```python
from build123d import *

# Parameters (mm, degrees)
SKETCH1_W           = 38.1
SKETCH1_H           = 15.24
BOSS_EXTRUDE2_DEPTH = 30.48
SKETCH2_W           = 50.8
SKETCH2_H           = 15.24
BOSS_EXTRUDE3_DEPTH = 38.1
SKETCH3_W           = 38.1
SKETCH3_H           = 17.78
CUT_EXTRUDE1_DEPTH  = 75.703641143
FILLET1_R           = 5.08
FILLET2_R           = 7.62


with BuildPart() as part:
    # Sketch1 → Boss-Extrude2 (new body)
    with BuildSketch(Plane.XY):
        Rectangle(SKETCH1_W, SKETCH1_H)
    extrude(amount=BOSS_EXTRUDE2_DEPTH)

    # Sketch2 → Boss-Extrude3 (add)
    with BuildSketch(Plane.XY.offset(30.48)):
        Rectangle(SKETCH2_W, SKETCH2_H)
    extrude(amount=BOSS_EXTRUDE3_DEPTH)

    # Sketch3 → Cut-Extrude1 (cut, through all)
    with BuildSketch(Plane.XZ.offset(7.62)):
        with Locations((0, 47.494377682)):
            Rectangle(SKETCH3_W, SKETCH3_H)
    extrude(amount=-CUT_EXTRUDE1_DEPTH, mode=Mode.SUBTRACT)

    # Fillet1
    fillet1_edges = [part.edges().sort_by_distance(p)[0] for p in [
        (-19.05, 0, 38.604377682),
        (-19.05, 0, 56.384377682),
        (19.05, 0, 56.384377682),
        (19.05, 0, 38.604377682),
    ]]
    fillet(fillet1_edges, radius=FILLET1_R)

    # Fillet2
    # the kernel refuses this fillet: 7.62 mm, written as the material it takes off along each edge
    with BuildSketch(Plane(origin=(-25.4, 26.403553311, 30.48), x_dir=(0, 0, 1), z_dir=(0, -1, 0)), Plane(origin=(25.4, -26.403553311, 30.48), x_dir=(0, 0, 1), z_dir=(0, 1, 0))) as fillet2_piece_1:
        with BuildLine():
            CenterArc((7.513421325, -7.62), FILLET2_R, 90, 80.405931773)
            Line((0, -6.35), (-0.150268426, -6.3246))
            ThreePointArc((-0.150268426, -6.3246), (-0.1524, -3.175), (-0.1524, 0))
            Line((-0.1524, 0), (0, 0.1524))
            Line((0, 0.1524), (7.513421325, 0.1524))
            Line((7.513421325, 0.1524), (7.513421325, 0))
        make_face()
    extrude(amount=52.807106623, mode=Mode.SUBTRACT)
    with BuildSketch(Plane(origin=(25.4, -26.67, 68.58), x_dir=(-1, 0, 0), z_dir=(0, 1, 0))) as fillet2_piece_2:
        with BuildLine():
            CenterArc((FILLET2_R, -FILLET2_R), FILLET2_R, 90, 90)
            Line((0, -FILLET2_R), (-FILLET2_R * 0.02, -FILLET2_R))
            Line((-FILLET2_R * 0.02, -FILLET2_R), (-FILLET2_R * 0.02, FILLET2_R * 0.02))
            Line((-FILLET2_R * 0.02, FILLET2_R * 0.02), (FILLET2_R, FILLET2_R * 0.02))
            Line((FILLET2_R, FILLET2_R * 0.02), (FILLET2_R, 0))
        make_face()
    extrude(amount=53.34, mode=Mode.SUBTRACT)
    with BuildSketch(Plane(origin=(-25.4, 26.67, 68.58), x_dir=(0, 0, -1), z_dir=(0, -1, 0))) as fillet2_piece_3:
        with BuildLine():
            CenterArc((FILLET2_R, FILLET2_R), FILLET2_R, 180, 90)
            Line((0, FILLET2_R), (-FILLET2_R * 0.02, FILLET2_R))
            Line((-FILLET2_R * 0.02, FILLET2_R), (-FILLET2_R * 0.02, -FILLET2_R * 0.02))
            Line((-FILLET2_R * 0.02, -FILLET2_R * 0.02), (FILLET2_R, -FILLET2_R * 0.02))
            Line((FILLET2_R, -FILLET2_R * 0.02), (FILLET2_R, 0))
        make_face()
    extrude(amount=53.34, mode=Mode.SUBTRACT)


solid = part.part
```
Geometry check sheet. Reference: the model listing, model coordinates, mm. A direction names the side the tool comes from. Round coordinates to 2 decimals unless told otherwise and drop trailing zeros. Loops run counter-clockwise (first coordinate to the right, second up) from the corner with the lowest first, then second, coordinate; pieces in that order, holes last. Notation, with made-up numbers: (21, 5.5) - (75, 5.5) arc R26 ccw to (75, 38.5) - close; hole circle Ø8 at (-25, -0.5). An arc over 180 degrees is marked (long way). Write each question's results on one line, items separated by ' | '. Start each with the question number.
Q1. Release check for a two-part mould opening along X. For faces 1 (the cylindrical face through (-23.109, 0.107, 66.407)), 2 (the flat face through (0, 7.62, 34)), 3 (the flat face through (-19.05, 0, 47)) record: +X half, -X half, draft (parallel to the pull), parting line (faces both ways), or undercut.
Q2. Cross-section at C-C on y = -0.25. Enter the section's corners in (x, z).
Q3. Thickness scan on line 1 (Z direction, x = 6.5, y = 1.25); line 2 (X direction, y = -5.5, z = 45); line 3 (X direction, y = -7, z = 53). Record the ranges inside material, lowest first. Write a range as [from, to].
Q4. Cross-section at B-B on z = 48.5. Enter the section's corners in (x, y).
Q5. Gauge pin test, flat ends, axial feed: P1, Ø5, axis at x = 7, z = 43.5, coming from the -Y side; P2, Ø8, axis at y = -5.5, z = 8, coming from the -X side. Record the tip position at first contact, or that the pin passes through.
Q6. Access from +Z, -Z, +X, -X, +Y, -Y to the whole of each face (thin tool, end or side, straight path). Record for faces 4 (the cylindrical face through (23.109, -0.107, 66.407)), 5 (the flat face through (-19.05, 0, 15)), 6 (the flat face through (0, 0, 38.604)).
Q7. Cross-section at A-A on x = -0.5. Enter the section's corners in (y, z), and give its area (3 significant figures).
Q8. Cross-section at D-D on z = 15.5. Enter the section's corners in (x, y).
Answers below:
1) face 1: -X half | face 2: draft | face 3: undercut
2) outline: (-25.4, 37.99) arc R7.62 ccw to (-19.05, 30.48) - (-19.05, 0) - (19.05, 0) - (19.05, 30.48) arc R7.62 ccw to (25.4, 37.99) - (25.4, 60.96) arc R7.62 ccw to (17.78, 68.58) - (-17.78, 68.58) arc R7.62 ccw to (-25.4, 60.96) - close; hole (-19.05, 43.68) arc R5.08 ccw to (-13.97, 38.6) - (13.97, 38.6) arc R5.08 ccw to (19.05, 43.68) - (19.05, 51.3) arc R5.08 ccw to (13.97, 56.38) - (-13.97, 56.38) arc R5.08 ccw to (-19.05, 51.3) - close
3) line 1: z = [0, 38.6], [56.38, 68.58] | line 2: x = [-25.4, -19.05], [19.05, 25.4] | line 3: x = [-25.4, -18.76], [18.76, 25.4]
4) outline: (-25.4, -7.62) - (-19.05, -7.62) - (-19.05, 7.62) - (-25.4, 7.62) - close; (19.05, -7.62) - (25.4, -7.62) - (25.4, 7.62) - (19.05, 7.62) - close
5) P1: passes through | P2: stops at x = -19.05
6) face 4: +Z, +X, +Y, -Y | face 5: -Z, -X, +Y, -Y | face 6: +Y, -Y
7) outline: (-7.62, 0) - (7.62, 0) - (7.62, 38.6) - (-7.62, 38.6) - close; (-7.62, 56.38) - (7.62, 56.38) - (7.62, 68.58) - (-7.62, 68.58) - close | area: 774 mm²
8) outline: (-19.05, -7.62) - (19.05, -7.62) - (19.05, 7.62) - (-19.05, 7.62) - close
